from build123d import *

# Parameters (mm, degrees)
SKETCH1_W                 = 55
SKETCH1_H                 = 75
SKETCH1_W_2               = 24.25
SKETCH1_H_2               = 11
BOSS_EXTRUDE1_DEPTH       = 4.5
SKETCH2_R                 = 1.45
SCREWHOLES_DEPTH          = 47.719910103
SKETCH4_W                 = 9.6
SKETCH4_H                 = 4.3
MOUNTINGPLATETAB_DEPTH    = 47.719910103
SKETCH5_R                 = 1.45
SKETCH5_W                 = 4.3
SKETCH5_H                 = 9.6
BRACETABS_DEPTH           = 47.719910103
SKETCH8_R                 = 1.45
EXPANSIONSCREWHOLES_DEPTH = 47.719910103
CABLETIESLOT_DEPTH        = 47.719910103


with BuildPart() as part:
    # Sketch1 → Boss-Extrude1 (new body)
    with BuildSketch(Plane.XY):
        Rectangle(SKETCH1_W, SKETCH1_H)
        with Locations((-13.375, 22.5)):
            Rectangle(SKETCH1_W_2, SKETCH1_H_2, mode=Mode.SUBTRACT)
        with Locations((13.375, 22.5)):
            Rectangle(SKETCH1_W_2, SKETCH1_H_2, mode=Mode.SUBTRACT)
        with Locations((13.375, -22.5)):
            Rectangle(SKETCH1_W_2, SKETCH1_H_2, mode=Mode.SUBTRACT)
        with Locations((-13.375, -22.5)):
            Rectangle(SKETCH1_W_2, SKETCH1_H_2, mode=Mode.SUBTRACT)
    extrude(amount=BOSS_EXTRUDE1_DEPTH)

    # Sketch2 → screwHoles (cut, through all)
    with BuildSketch(Plane.XY.offset(4.5)):
        with Locations((-15, 33)):
            Circle(SKETCH2_R)
        with Locations(Location((15, 33, 0), (0, 0, 180))):
            Circle(SKETCH2_R)
        with Locations((15, 0)):
            Circle(SKETCH2_R)
        with Locations(Location((-15, 0, 0), (0, 0, 180))):
            Circle(SKETCH2_R)
    extrude(amount=-SCREWHOLES_DEPTH, mode=Mode.SUBTRACT)

    # Sketch4 → mountingPlateTab (cut, through all)
    with BuildSketch(Plane.XY.offset(4.5)):
        Rectangle(SKETCH4_W, SKETCH4_H)
    extrude(amount=-MOUNTINGPLATETAB_DEPTH, mode=Mode.SUBTRACT)

    # Sketch5 → BraceTabs (cut, through all)
    with BuildSketch(Plane.XY.offset(4.5)):
        with Locations((23, -31.75)):
            Circle(SKETCH5_R)
        with Locations(Location((-23, -31.75, 0), (0, 0, 180))):
            Circle(SKETCH5_R)
        with Locations((23, -9.75)):
            Rectangle(SKETCH5_W, SKETCH5_H)
        with Locations((-23, -9.75)):
            Rectangle(SKETCH5_W, SKETCH5_H)
    extrude(amount=-BRACETABS_DEPTH, mode=Mode.SUBTRACT)

    # Sketch8 → ExpansionScrewholes (cut, through all)
    with BuildSketch(Plane.XY.offset(4.5)):
        with Locations((-15, -12)):
            Circle(SKETCH8_R)
        with Locations(Location((15, -12, 0), (0, 0, 180))):
            Circle(SKETCH8_R)
    extrude(amount=-EXPANSIONSCREWHOLES_DEPTH, mode=Mode.SUBTRACT)

    # Sketch12 → CableTieSlot (cut, through all)
    with BuildSketch(Plane.XY.offset(4.5)):
        with BuildLine():
            Line((-2.5, 34.5), (2.5, 34.5))
            ThreePointArc((2.5, 34.5), (3.5, 33.5), (2.5, 32.5))
            Line((2.5, 32.5), (-2.5, 32.5))
            ThreePointArc((-2.5, 32.5), (-3.5, 33.5), (-2.5, 34.5))
        make_face()
    extrude(amount=-CABLETIESLOT_DEPTH, mode=Mode.SUBTRACT)


solid = part.part
The model under review builds one solid part; all positions refer to its coordinate system, in mm. A direction names the side the tool comes from. Give positions to 0.01 mm unless a question says otherwise; leave off trailing zeros. Order: outer loops, then holes, each group sorted by start corner. A loop starts at its lowest first (then second) coordinate and runs counter-clockwise, first axis right, second up. Notation, with made-up numbers: (-20, 2.25) -> (2, 2.25) arc R10 ccw to (2, 18.25) -> close; hole circle Ø1 at (24.25, 74.25). An arc over 180 degrees is marked (long way). Write item = value, one per line. Start each with the question number.
(1) Draft analysis for pull direction Y (two halves, no side actions). For faces 1 (the flat face through (0, -8, 4.5)), 2 (the cylindrical face through (-16.38, -0.44, 2.28)), 3 (the flat face through (0, -37.5, 2)), state which applies: +Y half, -Y half, draft (parallel to the pull), parting line (faces both ways), or undercut.
(2) Take a section at D-D (z = 3.1). State how many separate pieces and enclosed holes the cut face has, plus the area to 3 significant figures.
(3) Take a section at C-C (x = -23). Write out the cut boundary in (y, z), plus the area to 3 significant figures.
(4) Tool access review of faces 4 (the flat face through (0, 37.5, 2)), 5 (the cylindrical face through (3.5, 33.5, 2.3)): name each direction out of +Z, -Z, +X, -X, +Y, -Y from which nothing blocks a thin tool from reaching the whole face with its end or side.
(5) Take a section at B-B (y = 26). Write out the cut boundary in (x, z).
(6) Take a section at A-A (x = 15). Write out the cut boundary in (y, z).
(7) For L1, parallel to Y at x = -25, z = 3.7; L2, parallel to X at y = -24, z = 1.7; L3, parallel to Y at x = 17, z = 0.4, list the stretches that pass through material, from the lowest coordinate up. Write a range as from..to.
(8) For pin 1 Ø2.5 at (x, y) = (23, -31.75) entering from +Z, flat-tipped, find the tip position at first contact; note if it passes through.
Returned:
q1.face_1 = draft
q1.face_2 = undercut
q1.face_3 = -Y half
q2.separate_pieces = 1
q2.enclosed_holes = 16
q2.area = 2,870 mm²
q3.outline = (-37.5, 0) -> (-33.2, 0) -> (-33.2, 4.5) -> (-37.5, 4.5) -> close; (-30.3, 0) -> (-28, 0) -> (-28, 4.5) -> (-30.3, 4.5) -> close; (-17, 0) -> (-14.55, 0) -> (-14.55, 4.5) -> (-17, 4.5) -> close; (-4.95, 0) -> (17, 0) -> (17, 4.5) -> (-4.95, 4.5) -> close; (28, 0) -> (37.5, 0) -> (37.5, 4.5) -> (28, 4.5) -> close
q3.area = 182 mm²
q4.face_4 = +Z, -Z, +X, -X, +Y
q4.face_5 = +Z, -Z
q5.outline = (-27.5, 0) -> (-25.5, 0) -> (-25.5, 4.5) -> (-27.5, 4.5) -> close; (-1.25, 0) -> (1.25, 0) -> (1.25, 4.5) -> (-1.25, 4.5) -> close; (25.5, 0) -> (27.5, 0) -> (27.5, 4.5) -> (25.5, 4.5) -> close
q6.outline = (-37.5, 0) -> (-28, 0) -> (-28, 4.5) -> (-37.5, 4.5) -> close; (-17, 0) -> (-13.45, 0) -> (-13.45, 4.5) -> (-17, 4.5) -> close; (-10.55, 0) -> (-1.45, 0) -> (-1.45, 4.5) -> (-10.55, 4.5) -> close; (1.45, 0) -> (17, 0) -> (17, 4.5) -> (1.45, 4.5) -> close; (28, 0) -> (31.55, 0) -> (31.55, 4.5) -> (28, 4.5) -> close; (34.45, 0) -> (37.5, 0) -> (37.5, 4.5) -> (34.45, 4.5) -> close
q7.L1 = -37.5..-28, -17..-14.55, -4.95..17, 28..37.5
q7.L2 = -27.5..-25.5, -1.25..1.25, 25.5..27.5
q7.L3 = -37.5..-28, -17..17, 28..37.5
q8.pin_1 = through
